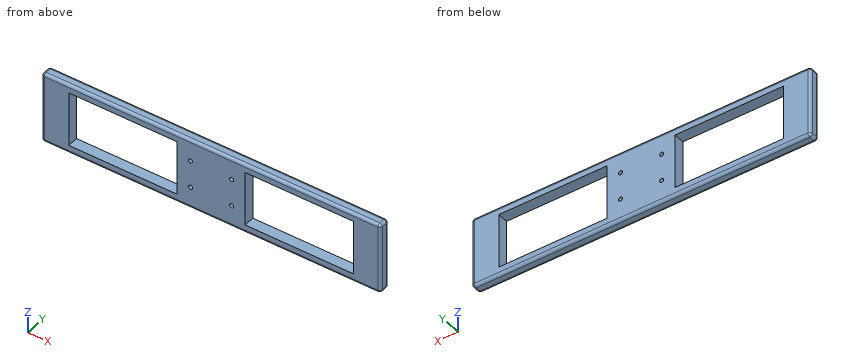
```python
from build123d import *

# Parameters (mm, degrees)
SKETCH1_W                 = 125
SKETCH1_H                 = 26
BOSS_EXTRUDE1_DEPTH       = 4
SKETCH2_W                 = 40
SKETCH2_H                 = 20
CUT_EXTRUDE1_DEPTH        = 4
FILLET5_R                 = 1
F_1_5MM_DOWEL_HOLE1_D     = 1.5
F_1_5MM_DOWEL_HOLE1_DEPTH = 8
F_1_5MM_DOWEL_HOLE1_TIP   = 0.450645464


with BuildPart() as part:
    # Sketch1 → Boss-Extrude1 (new body)
    with BuildSketch(Plane(origin=(0, 0, 0), x_dir=(1, 0, 0), z_dir=(0, 1, 0))):
        with Locations((62.5, 13)):
            Rectangle(SKETCH1_W, SKETCH1_H)
    extrude(amount=BOSS_EXTRUDE1_DEPTH)

    # Sketch2 → Cut-Extrude1 (cut)
    with BuildSketch(Plane(origin=(0, 4, 0), x_dir=(1, 0, 0), z_dir=(0, 1, 0))):
        with Locations((30, 13)):
            Rectangle(SKETCH2_W, SKETCH2_H)
        with Locations((95, 13)):
            Rectangle(SKETCH2_W, SKETCH2_H)
    extrude(amount=-CUT_EXTRUDE1_DEPTH, mode=Mode.SUBTRACT)

    # Fillet5
    fillet5_edges = [part.edges().sort_by_distance(p)[0] for p in [
        (125, 4, -13),
        (62.5, 4, -26),
        (0, 4, -13),
        (62.5, 0, -26),
        (125, 0, -13),
        (62.5, 0, 0),
        (0, 0, -13),
        (0, 2, -26),
        (125, 2, -26),
        (125, 2, 0),
        (0, 2, 0),
        (62.5, 4, 0),
    ]]
    fillet(fillet5_edges, radius=FILLET5_R)

    # Ø1.5mm Dowel Hole1
    with Locations(Plane(origin=(0, 4, 0), x_dir=(1, 0, 0), z_dir=(0, 1, 0))):
        with Locations((54.9, 8), (54.9, 18), (70.1, 18), (70.1, 8)):
            Hole(F_1_5MM_DOWEL_HOLE1_D / 2, depth=F_1_5MM_DOWEL_HOLE1_DEPTH)
            with Locations((0, 0, -(F_1_5MM_DOWEL_HOLE1_DEPTH + F_1_5MM_DOWEL_HOLE1_TIP / 2))):  # 118° drill point
                Cone(0, F_1_5MM_DOWEL_HOLE1_D / 2, F_1_5MM_DOWEL_HOLE1_TIP, mode=Mode.SUBTRACT)


solid = part.part
```
Input: part model. Units: mm. Frame: model coordinates. Round coordinates to 2 decimals unless told otherwise and drop trailing zeros. Order: outer loops, then holes, each group sorted by start corner. A loop starts at its lowest first (then second) coordinate and runs counter-clockwise, first axis right, second up. Notation, with made-up numbers: (-12.5, -20.75) - (41.5, -20.75) arc R22 ccw to (41.5, 11.25) - close; hole circle Ø9 at (43.5, 35). An arc over 180 degrees is marked (long way). One line per question, with ' | ' between items. Start each with the question number.
1) Cut plane B-B, the plane z = -4.75. Return the cut outline in (x, y), then the cut area to 3 significant figures.
2) Ray query, probe 1 along Z at (x, y) = (70.1, 1.5); probe 2 along X at (y, z) = (1.5, -21); probe 3 along X at (y, z) = (2.6, -8). Return the intervals inside material, ascending.
3) Cut plane A-A, the plane y = 1.75. Return the cut outline in (x, z), then the cut area to 3 significant figures.
4) Cut plane C-C, the plane x = 112. Return the cut outline in (y, z), then the cut area to 3 significant figures.
Worked out:
1) outline: (0, 1) arc R1 ccw to (1, 0) - (10, 0) - (10, 4) - (1, 4) arc R1 ccw to (0, 3) - close; (50, 0) - (75, 0) - (75, 4) - (50, 4) - close; (115, 0) - (124, 0) arc R1 ccw to (125, 1) - (125, 3) arc R1 ccw to (124, 4) - (115, 4) - close | area: 179 mm^2
2) probe 1: z = -26 to -18.75, -17.25 to -8.75, -7.25 to 0 | probe 2: x = 0 to 10, 50 to 75, 115 to 125 | probe 3: x = 0 to 10, 50 to 54.15, 55.65 to 69.35, 70.85 to 75, 115 to 125
3) outline: (0, -25) arc R1 ccw to (1, -26) - (124, -26) arc R1 ccw to (125, -25) - (125, -1) arc R1 ccw to (124, 0) - (1, 0) arc R1 ccw to (0, -1) - close; hole (10, -23) - (50, -23) - (50, -3) - (10, -3) - close; hole circle Ø1.5 at (54.9, -18); hole circle Ø1.5 at (54.9, -8); hole circle Ø1.5 at (70.1, -18); hole circle Ø1.5 at (70.1, -8); hole (75, -23) - (115, -23) - (115, -3) - (75, -3) - close | area: 1,640 mm^2
4) outline: (0, -25) arc R1 ccw to (1, -26) - (3, -26) arc R1 ccw to (4, -25) - (4, -23) - (0, -23) - close; (0, -3) - (4, -3) - (4, -1) arc R1 ccw to (3, 0) - (1, 0) arc R1 ccw to (0, -1) - close | area: 23.1 mm^2
